```python
from build123d import *

# Parameters (mm, degrees)
BOX002_W       = 32
BOX002_H       = 2
BOX002_DEPTH   = 5
BOX001_W       = 32
BOX001_H       = 2
BOX001_DEPTH   = 5
BOX_W          = 35
BOX_H          = 19
BOX_DEPTH      = 10
FILLET001_R    = 1
BOX003_W       = 36
BOX003_H       = 20
BOX003_DEPTH   = 10
FILLET002_R    = 2
BOX005_W       = 6
BOX005_H       = 21
BOX005_DEPTH   = 3
BOX004_W       = 4
BOX004_H       = 25
BOX004_DEPTH   = 5
CYLINDER_R     = 9
CYLINDER_DEPTH = 8
FILLET_R       = 2


with BuildPart() as box002:
    # Box002 → Box002 (new body)
    with BuildSketch(Plane(origin=(-1, 17.5, 5), x_dir=(1, 0, 0), z_dir=(0, 0, 1))):
        with Locations((16, 1)):
            Rectangle(BOX002_W, BOX002_H)
    extrude(amount=BOX002_DEPTH)


with BuildPart() as fusion:
    # Box001 → Box001 (new body)
    with BuildSketch(Plane(origin=(-1, -0.5, 5), x_dir=(1, 0, 0), z_dir=(0, 0, 1))):
        with Locations((16, 1)):
            Rectangle(BOX001_W, BOX001_H)
    extrude(amount=BOX001_DEPTH)

    # Fusion: union Box002
    add(box002.part)


with BuildPart() as fillet001:
    # Box → Box (new body)
    with BuildSketch(Plane.XY):
        with Locations((17.5, 9.5)):
            Rectangle(BOX_W, BOX_H)
    extrude(amount=BOX_DEPTH)

    # Cut: cut Fusion
    add(fusion.part, mode=Mode.SUBTRACT)

    # Fillet001
    fillet001_edges = [fillet001.edges().sort_by_distance(p)[0] for p in [
        (0, 0, 2.5),
        (0, 19, 2.5),
        (35, 0, 5),
        (35, 19, 5),
    ]]
    fillet(fillet001_edges, radius=FILLET001_R)


with BuildPart() as fillet002:
    # Box003 → Box003 (new body)
    with BuildSketch(Plane(origin=(-0.5, -0.5, 10), x_dir=(1, 0, 0), z_dir=(0, 0, 1))):
        with Locations((18, 10)):
            Rectangle(BOX003_W, BOX003_H)
    extrude(amount=BOX003_DEPTH)

    # Fillet002
    fillet002_edges = [fillet002.edges().sort_by_distance(p)[0] for p in [
        (-0.5, -0.5, 15),
        (-0.5, 9.5, 20),
        (-0.5, 19.5, 15),
        (35.5, -0.5, 15),
        (35.5, 9.5, 20),
        (35.5, 19.5, 15),
        (17.5, -0.5, 20),
        (17.5, 19.5, 20),
    ]]
    fillet(fillet002_edges, radius=FILLET002_R)


with BuildPart() as box005:
    # Box005 → Box005 (new body)
    with BuildSketch(Plane(origin=(30.5, -1, 7), x_dir=(1, 0, 0), z_dir=(0, 0, 1))):
        with Locations((3, 10.5)):
            Rectangle(BOX005_W, BOX005_H)
    extrude(amount=BOX005_DEPTH)


with BuildPart() as cut001:
    # Box004 → Box004 (new body)
    with BuildSketch(Plane(origin=(31.5, -3, 7.5), x_dir=(1, 0, 0), z_dir=(0, 0, 1))):
        with Locations((2, 12.5)):
            Rectangle(BOX004_W, BOX004_H)
    extrude(amount=BOX004_DEPTH)

    # Cut001: cut Box005
    add(box005.part, mode=Mode.SUBTRACT)


with BuildPart() as fusion001:
    # Cylinder → Cylinder (new body)
    with BuildSketch(Plane(origin=(35.5, 9.5, 10), x_dir=(0, 0, -1), z_dir=(1, 0, 0))):
        Circle(CYLINDER_R)
    extrude(amount=CYLINDER_DEPTH)

    # Fillet
    fillet_edges = [fusion001.edges().sort_by_distance(p)[0] for p in [
        (35.5, 9.5, 19),
    ]]
    fillet(fillet_edges, radius=FILLET_R)

    # Fusion001: union Fillet001, Fillet002, Cut001
    add(fillet001.part)
    add(fillet002.part)
    add(cut001.part)


solid = fusion001.part
```
Source: CAD feature listing. Evaluate the final solid. Frame: model axes, mm. A direction names the side the tool comes from. Round coordinates to 2 decimals unless told otherwise and drop trailing zeros. Loops run counter-clockwise (first coordinate to the right, second up) from the corner with the lowest first, then second, coordinate; pieces in that order, holes last. Notation, with made-up numbers: M -25,-26.75 L 34,-26.75 A17 cw 34,-17.75 Z; hole C 26.5,73 d10. An arc over 180 degrees is marked long. Use a Markdown table: item, result. Add a question column.
1. Contact query for flat-ended pins moving along their axis: pin 1 (1 mm diameter, centred on x = 8.5, z = 7.5, fed in from -Y); pin 2 (0.8 mm diameter, centred on y = 18.5, z = 6.5, fed in from -X); pin 3 (0.8 mm diameter, centred on y = -1.5, z = 10.5, fed in from -X). Output: stop coordinate, or through.
2. Ray query, line 1 along X through (y, z) = (8.75, 5.75); line 2 along Y through (x, z) = (2, 4); line 3 along Y through (x, z) = (26.5, 16.75). Return the intervals inside material, ascending. Write a range as [from, to].
3. Pull-direction query (X, two-part tool) for faces 4 (the flat face through (15, 17.5, 7)), 5 (the cylindrical face through (34.93, 9.61, 19.4)), 6 (the cylindrical face through (0.285, 0.301, 2.535)); classes: +X half, -X half, draft (parallel to the pull), parting line (faces both ways), or undercut.
4. Cut plane A-A, the plane y = 9.5. Output: boundary loops of the cut face in (x, z).
5. Cut plane B-B, the plane x = 9. Output: boundary loops of the cut face in (y, z), and give its area (3 significant figures).
6. Set-up query: faces 1 (the cylindrical face through (0.285, 18.699, 2.535)), 2 (the flat face through (33, 20, 9)), 3 (the cylindrical face through (40.458, 0.714, 11.951)). Return all of +Z, -Z, +X, -X, +Y, -Y with unobstructed straight access to the full face (end or side cutting, diameter ignored); none if empty.
Solution:
| question | item | result |
|---|---|---|
| 1 | pin 1 | stops at y = 1.5 |
| 1 | pin 2 | stops at x = 31 |
| 1 | pin 3 | stops at x = 31.5 |
| 2 | line 1 | x = [0, 35], [35.5, 43.5] |
| 2 | line 2 | y = [0, 19] |
| 2 | line 3 | y = [-0.5, 19.5] |
| 3 | face 4 | draft |
| 3 | face 5 | undercut |
| 3 | face 6 | -X half |
| 4 | outline | M -0.5,10 L 0,10 L 0,0 L 35,0 L 35,10 L 35.5,10 L 35.5,3 A2 ccw 37.5,1 L 43.5,1 L 43.5,19 L 37.5,19 A2 ccw 35.5,17 L 35.5,18 A2 ccw 33.5,20 L 1.5,20 A2 ccw -0.5,18 Z |
| 5 | outline | M -0.5,10 L 1.5,10 L 1.5,5 L 0,5 L 0,0 L 19,0 L 19,5 L 17.5,5 L 17.5,10 L 19.5,10 L 19.5,18 A2 ccw 17.5,20 L 1.5,20 A2 ccw -0.5,18 Z |
| 5 | area | 373 mm2 |
| 6 | face 1 | -Z, -X, +Y |
| 6 | face 2 | -Z, +X, -X |
| 6 | face 3 | +X |
